from build123d import *

# Parameters (mm, degrees)
SKETCH1_R           = 25
SKETCH1_R_2         = 2
BOSS_EXTRUDE1_DEPTH = 5
SKETCH2_R           = 12.5
SKETCH2_R_2         = 7.5
BOSS_EXTRUDE2_DEPTH = 10


with BuildPart() as part:
    # Sketch1 → Boss-Extrude1 (new body)
    with BuildSketch(Plane.XY):
        Circle(SKETCH1_R)
        with Locations((0, 20)):
            Circle(SKETCH1_R_2, mode=Mode.SUBTRACT)
        with Locations((17.320508076, 10)):
            Circle(SKETCH1_R_2, mode=Mode.SUBTRACT)
        with Locations((17.320508076, -10)):
            Circle(SKETCH1_R_2, mode=Mode.SUBTRACT)
        with Locations((0, -20)):
            Circle(SKETCH1_R_2, mode=Mode.SUBTRACT)
        with Locations((-17.320508076, -10)):
            Circle(SKETCH1_R_2, mode=Mode.SUBTRACT)
        with Locations((-17.320508076, 10)):
            Circle(SKETCH1_R_2, mode=Mode.SUBTRACT)
    extrude(amount=BOSS_EXTRUDE1_DEPTH)

    # Sketch2 → Boss-Extrude2 (add)
    with BuildSketch(Plane.XY.offset(5)):
        Circle(SKETCH2_R)
        Circle(SKETCH2_R_2, mode=Mode.SUBTRACT)
    extrude(amount=BOSS_EXTRUDE2_DEPTH)


solid = part.part
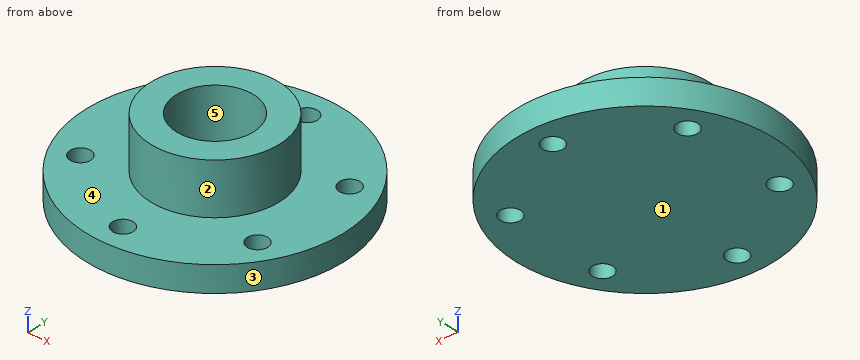
CAD build for the part. Positions are in the model's coordinates, mm. Face numbers are marked on the shaded views. A direction names the side the tool comes from. Give positions to 0.01 mm unless a question says otherwise; leave off trailing zeros. Order: outer loops, then holes, each group sorted by start corner. A loop starts at its lowest first (then second) coordinate and runs counter-clockwise, first axis right, second up. Notation, with made-up numbers: (2, -14.5) -> (7, -14.5) arc R33 ccw to (7, 23.5) -> close; hole circle Ø5 at (4.25, 51.25). An arc over 180 degrees is marked (long way). Return JSON: item names as keys, results as strings.
Q1. Which spindle directions (+Z, -Z, +X, -X, +Y, -Y) get a long thin tool onto all of the face, cutting with end or side? Do the marked faces 1 and 2. Say none if no direction does.
Working result:
{"face 1": "-Z, +X, -X, +Y, -Y", "face 2": "+Z"}
Q2. Drill centre lines: line 1 (Y direction, x = 0, z = 3.25); line 2 (Y direction, x = -6, z = 11.75); line 3 (Y direction, x = 1, z = 6.75). Where is each one in solid material? Low to high.
Working result:
{"line 1": "-25 to -22, -18 to 18, 22 to 25", "line 2": "-10.97 to -4.5, 4.5 to 10.97", "line 3": "-12.46 to -7.43, 7.43 to 12.46"}
Q3. Saw through at A-A (y = -20). Write the cut outline in (x, z), then the cut area to 3 significant figures.
Working result:
{"outline": "(-15, 0) -> (-2, 0) -> (-2, 5) -> (-15, 5) -> close; (2, 0) -> (15, 0) -> (15, 5) -> (2, 5) -> close", "area": "130 mm²"}
Q4. Saw through at D-D (y = -10). Write the cut outline in (x, z).
Working result:
{"outline": "(-22.91, 0) -> (-19.32, 0) -> (-19.32, 5) -> (-22.91, 5) -> close; (-15.32, 0) -> (15.32, 0) -> (15.32, 5) -> (7.5, 5) -> (7.5, 15) -> (-7.5, 15) -> (-7.5, 5) -> (-15.32, 5) -> close; (19.32, 0) -> (22.91, 0) -> (22.91, 5) -> (19.32, 5) -> close"}
Q5. Flat gauge pins, fed straight in: pin 1 (4.5 mm diameter, centred on x = 17.32, y = 10, fed in from +Z); pin 2 (1 mm diameter, centred on y = -15, z = 2.5, fed in from +X); pin 3 (4 mm diameter, centred on y = -2, z = 10.5, fed in from -X). Where does each tip first touch, or does it go through?
Working result:
{"pin 1": "z = 5", "pin 2": "x = 20.37", "pin 3": "x = -12.5"}
Q6. Saw through at C-C (z = 4.25). Write the cut outline in (x, y).
Working result:
{"outline": "circle Ø50 at (0, 0); hole circle Ø4 at (-17.32, -10); hole circle Ø4 at (-17.32, 10); hole circle Ø4 at (0, -20); hole circle Ø4 at (0, 20); hole circle Ø4 at (17.32, -10); hole circle Ø4 at (17.32, 10)"}
Q7. Saw through at B-B (x = 0). Write the cut outline in (y, z), then the cut area to 3 significant figures.
Working result:
{"outline": "(-25, 0) -> (-22, 0) -> (-22, 5) -> (-25, 5) -> close; (-18, 0) -> (18, 0) -> (18, 5) -> (12.5, 5) -> (12.5, 15) -> (7.5, 15) -> (7.5, 5) -> (-7.5, 5) -> (-7.5, 15) -> (-12.5, 15) -> (-12.5, 5) -> (-18, 5) -> close; (22, 0) -> (25, 0) -> (25, 5) -> (22, 5) -> close", "area": "310 mm²"}
Q8. Mould opens along X. For the marked faces 3, 4 and 5 say: pulls with the +X half, pulls with the -X half, needs draft (parallel to the pull), parting line crosses it, or undercut.
Working result:
{"face 3": "parting line crosses it", "face 4": "needs draft", "face 5": "undercut"}
